Source: three-view drawing plus pictorial views. Frame: mm from the lowest corner of the part. Coordinates: 2 decimals unless noted, no trailing zeros. Loops run counter-clockwise (first coordinate to the right, second up) from the corner with the lowest first, then second, coordinate; pieces in that order, holes last. Notation, with made-up numbers: (0, 47) - (46, 47) arc R18 ccw to (46, 74) - close; hole circle Ø7 at (25, 26). An arc over 180 degrees is marked (long way). Return JSON: item names as keys, results as strings.
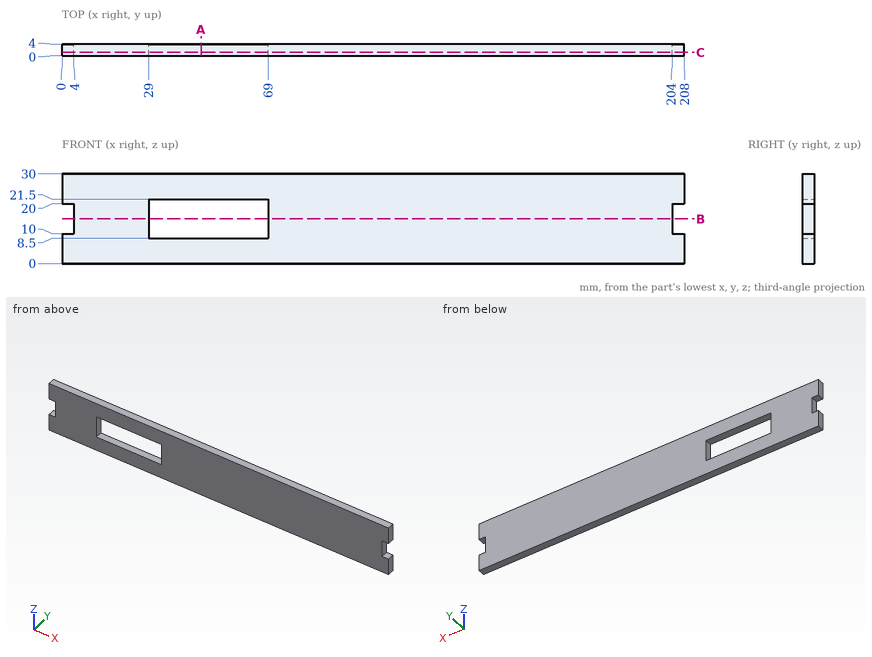
Item 1: Section query B-B, the plane z = 15. Return loops of the section in (x, y), and give its area (3 significant figures).
Worked out:
{"outline": "(4, 0) - (29, 0) - (29, 4) - (4, 4) - close; (69, 0) - (204, 0) - (204, 4) - (69, 4) - close", "area": "640 mm^2"}
Item 2: Section query C-C, the plane y = 1.2. Return loops of the section in (x, z).
Worked out:
{"outline": "(0, 0) - (208, 0) - (208, 10) - (204, 10) - (204, 20) - (208, 20) - (208, 30) - (0, 30) - (0, 20) - (4, 20) - (4, 10) - (0, 10) - close; hole (29, 8.5) - (69, 8.5) - (69, 21.5) - (29, 21.5) - close"}
Item 3: Section query A-A, the plane x = 46.5. Return loops of the section in (y, z).
Worked out:
{"outline": "(0, 0) - (4, 0) - (4, 8.5) - (0, 8.5) - close; (0, 21.5) - (4, 21.5) - (4, 30) - (0, 30) - close"}
Item 4: Ray query, probe 1 along X at (y, z) = (2.1, 14); probe 2 along Z at (x, y) = (31, 1.65). Return the intervals inside material, ascending. Write a range as from..to.
Worked out:
{"probe 1": "4..29, 69..204", "probe 2": "0..8.5, 21.5..30"}
Item 5: First-contact query: pin 1 Ø2 at (y, z) = (2, 16.5) entering from -X; pin 2 Ø1.2 at (y, z) = (1, 17.5) entering from +X. Flat tips, straight axial feed; report the tip coordinate or a pass-through.
Worked out:
{"pin 1": "x = 4", "pin 2": "x = 204"}
